Geometry check sheet. Reference: the model listing, model coordinates, mm. Give positions to 0.01 mm unless a question says otherwise; leave off trailing zeros. Write each loop counter-clockwise with the first axis right and the second up, starting at its lowest first coordinate (ties: lowest second). Pieces come first, ordered by that corner, then holes. Notation, with made-up numbers: M 75.5,41 L 103.5,41 A10 ccw 103.5,51 Z; hole C -10.5,-17 d10. An arc over 180 degrees is marked long. One line per item, written item: value. Start each with the question number.
1. Scan line: line 1 (Z direction, x = -24, y = -9). Record every from-to range of solid material in increasing order.
2. Gauge pin test, flat end, axial feed: pin 1 (12 mm diameter, centred on x = 21, y = 6, fed in from -Z). Record the tip position at first contact, or that the pin passes through.
3. Cross-section at B-B on x = 35.5. Record the cut outline in (y, z).
4. Cross-section at A-A on y = -5.5. Record the cut outline in (x, z), then the cut area to 3 significant figures.
5. Release check for a two-part mould opening along Z. For faces 1 (the face through (10, -3, 70)), 2 (the face through (10, -22.931, 143)), 3 (the face through (10, -3, 180)) record: pulls with the +Z half, pulls with the -Z half, needs draft (parallel to the pull), parting line crosses it, or undercut.
6. Cross-section at C-C on z = 103.5. Record the cut outline in (x, y), then the cut area to 3 significant figures.
from build123d import *

# Parameters (mm, degrees)
F0_W     = 90
F0_H     = 40
F1_DEPTH = 180
F2_W     = 86
F2_H     = 34
F3_DEPTH = 40.001
F4_W     = 36
F4_H     = 34
F5_DEPTH = 90.001


with BuildPart() as f1:
    # F0 (on Top) → F1 (new body)
    with BuildSketch(Plane.XY):
        with Locations((10.468276, -2.930649)):
            Rectangle(F0_W, F0_H)
    extrude(amount=F1_DEPTH)

    # F2 (on face) → F3 (cut, through all)
    with BuildSketch(Plane.XZ.offset(22.930649)):
        with Locations((10.468276, 161)):
            Rectangle(F2_W, F2_H)
        with Locations((10.468276, 125)):
            Rectangle(F2_W, F2_H)
        with Locations((10.468276, 89)):
            Rectangle(F2_W, F2_H)
        with Locations((10.468276, 53)):
            Rectangle(F2_W, F2_H)
        with Locations((10.468276, 17)):
            Rectangle(F2_W, F2_H)
    extrude(amount=-F3_DEPTH, mode=Mode.SUBTRACT)

    # F4 (on face) → F5 (cut, through all)
    with BuildSketch(Plane(origin=(-34.531724, 0, 0), x_dir=(0, -1, 0), z_dir=(-1, 0, 0))):
        with Locations((2.930649, 161)):
            Rectangle(F4_W, F4_H)
        with Locations((2.930649, 125)):
            Rectangle(F4_W, F4_H)
        with Locations((2.930649, 89)):
            Rectangle(F4_W, F4_H)
        with Locations((2.930649, 53)):
            Rectangle(F4_W, F4_H)
        with Locations((2.930649, 17)):
            Rectangle(F4_W, F4_H)
    extrude(amount=-F5_DEPTH, mode=Mode.SUBTRACT)


solid = f1.part
Report:
1. line 1: z = 34 to 36, 70 to 72, 106 to 108, 142 to 144, 178 to 180
2. pin 1: stops at z = 34
3. outline: M -22.93,34 L 17.07,34 L 17.07,36 L -22.93,36 Z; M -22.93,70 L 17.07,70 L 17.07,72 L -22.93,72 Z; M -22.93,106 L 17.07,106 L 17.07,108 L -22.93,108 Z; M -22.93,142 L 17.07,142 L 17.07,144 L -22.93,144 Z; M -22.93,178 L 17.07,178 L 17.07,180 L -22.93,180 Z
4. outline: M -34.53,34 L 55.47,34 L 55.47,36 L -34.53,36 Z; M -34.53,70 L 55.47,70 L 55.47,72 L -34.53,72 Z; M -34.53,106 L 55.47,106 L 55.47,108 L -34.53,108 Z; M -34.53,142 L 55.47,142 L 55.47,144 L -34.53,144 Z; M -34.53,178 L 55.47,178 L 55.47,180 L -34.53,180 Z
4. area: 900 mm^2
5. face 1: undercut
5. face 2: needs draft
5. face 3: pulls with the +Z half
6. outline: M -34.53,-22.93 L -32.53,-22.93 L -32.53,-20.93 L -34.53,-20.93 Z; M -34.53,15.07 L -32.53,15.07 L -32.53,17.07 L -34.53,17.07 Z; M 53.47,-22.93 L 55.47,-22.93 L 55.47,-20.93 L 53.47,-20.93 Z; M 53.47,15.07 L 55.47,15.07 L 55.47,17.07 L 53.47,17.07 Z
6. area: 16.0 mm^2
